Could you check a few things on this model? Use its own coordinates, in mm. Face numbers are marked on the shaded views. A direction names the side the tool comes from. Give positions to 0.01 mm unless a question says otherwise; leave off trailing zeros. Loops run counter-clockwise (first coordinate to the right, second up) from the corner with the lowest first, then second, coordinate; pieces in that order, holes last. Notation, with made-up numbers: (52, -1.5) - (97, -1.5) arc R20 cw to (97, 11.5) - close; hole circle Ø4 at (75.5, -20). An arc over 180 degrees is marked (long way). Write each question's results on one line, items separated by ' | '. Start each with the question number.
1) I want a section at D-D, the plane z = -22.75. Write out the boundary of the cut face in (x, y), and give its area (3 significant figures).
2) I want a section at A-A, the plane x = 25. Write out the boundary of the cut face in (y, z).
3) If we mould it in two halves opening along Z, with no side actions, what happens to the marked faces 1, 2 and 3? For each: +Z half, -Z half, draft (parallel to the pull), parting line (faces both ways), or undercut.
4) If I drill on probe 1 along X at (y, z) = (1.85, -7.5); probe 2 along X at (y, z) = (1.7, -6); probe 3 along Z at (x, y) = (4, 0.6), over which ranges is the centre line in solid material (lowest first)? Write a range as [from, to].
5) On a 3-axis mill with a long thin cutter (end or side, diameter ignored), from which of +Z, -Z, +X, -X, +Y, -Y can I reach the whole of each face in a straight line? I mean the marked faces 4 and 5. Say none if no direction works.
6) I want a section at B-B, the plane z = -17.5. Write out the boundary of the cut face in (x, y), and give its area (3 significant figures).
7) I want a section at C-C, the plane y = 1.55. Write out the boundary of the cut face in (x, z).
from build123d import *

# Parameters (mm, degrees)
SKETCH1_W           = 50
SKETCH1_H           = 25
SKETCH1_R           = 1.75
BOSS_EXTRUDE1_DEPTH = 3
SKETCH2_R           = 10
SKETCH2_W           = 10
SKETCH2_H           = 3
CUT_EXTRUDE1_DEPTH  = 10
FILLET1_R           = 5


with BuildPart() as part:
    # Sketch1 → Boss-Extrude1 (new body)
    with BuildSketch(Plane(origin=(0, 0, 0), x_dir=(1, 0, 0), z_dir=(0, 1, 0))):
        with Locations((25, 12.5)):
            Rectangle(SKETCH1_W, SKETCH1_H)
        with Locations(Location((25, 17.5, 0), (0, 0, 270))):
            Circle(SKETCH1_R, mode=Mode.SUBTRACT)
        with Locations(Location((25, 7.5, 0), (0, 0, 270))):
            Circle(SKETCH1_R, mode=Mode.SUBTRACT)
        with Locations(Location((5.463236706, 17.5, 0), (0, 0, 270))):
            Circle(SKETCH1_R, mode=Mode.SUBTRACT)
        with Locations(Location((5.463236706, 7.5, 0), (0, 0, 270))):
            Circle(SKETCH1_R, mode=Mode.SUBTRACT)
        with Locations(Location((44.777570027, 7.5, 0), (0, 0, 270))):
            Circle(SKETCH1_R, mode=Mode.SUBTRACT)
        with Locations(Location((44.777570027, 17.5, 0), (0, 0, 270))):
            Circle(SKETCH1_R, mode=Mode.SUBTRACT)
    extrude(amount=BOSS_EXTRUDE1_DEPTH)

    # Sketch2 → Cut-Extrude1 (cut)
    with BuildSketch(Plane(origin=(0, 3, 0), x_dir=(1, 0, 0), z_dir=(0, 1, 0))):
        with Locations((25, 32)):
            Circle(SKETCH2_R)
        with Locations((5, 23.5)):
            Rectangle(SKETCH2_W, SKETCH2_H)
        with Locations((45, 23.5)):
            Rectangle(SKETCH2_W, SKETCH2_H)
    extrude(amount=-CUT_EXTRUDE1_DEPTH, mode=Mode.SUBTRACT)

    # Fillet1
    # the kernel refuses this fillet: 5 mm, written as the material it takes off along each edge
    with BuildSketch(Plane(origin=(50, -12.5, 0), x_dir=(-1, 0, 0), z_dir=(0, 1, 0)), Plane(origin=(0, 15.5, -22), x_dir=(0, 0, 1), z_dir=(0, -1, 0))) as fillet1_piece_1:
        with BuildLine():
            CenterArc((FILLET1_R, -FILLET1_R), FILLET1_R, 90, 90)
            Line((0, -FILLET1_R), (-FILLET1_R * 0.02, -FILLET1_R))
            Line((-FILLET1_R * 0.02, -FILLET1_R), (-FILLET1_R * 0.02, FILLET1_R * 0.02))
            Line((-FILLET1_R * 0.02, FILLET1_R * 0.02), (FILLET1_R, FILLET1_R * 0.02))
            Line((FILLET1_R, FILLET1_R * 0.02), (FILLET1_R, 0))
        make_face()
    extrude(amount=28, mode=Mode.SUBTRACT)
    with BuildSketch(Plane(origin=(0, -12.5, 0), x_dir=(1, 0, 0), z_dir=(0, 1, 0)), Plane(origin=(50, 15.5, -22), x_dir=(0, 0, 1), z_dir=(0, -1, 0))) as fillet1_piece_2:
        with BuildLine():
            CenterArc((FILLET1_R, FILLET1_R), FILLET1_R, 180, 90)
            Line((0, FILLET1_R), (-FILLET1_R * 0.02, FILLET1_R))
            Line((-FILLET1_R * 0.02, FILLET1_R), (-FILLET1_R * 0.02, -FILLET1_R * 0.02))
            Line((-FILLET1_R * 0.02, -FILLET1_R * 0.02), (FILLET1_R, -FILLET1_R * 0.02))
            Line((FILLET1_R, -FILLET1_R * 0.02), (FILLET1_R, 0))
        make_face()
    extrude(amount=28, mode=Mode.SUBTRACT)
    with BuildSketch(Plane(origin=(40, 14.456439237, -25), x_dir=(-1, 0, 0), z_dir=(0, -1, 0))) as fillet1_piece_3:
        with BuildLine():
            CenterArc((4.582575695, -5), FILLET1_R, 90, 66.421821522)
            Line((0, -3), (-0.091651514, -2.96))
            ThreePointArc((-0.091651514, -2.96), (-0.1, -1.5), (-0.1, 0))
            Line((-0.1, 0), (0, 0.1))
            Line((0, 0.1), (4.582575695, 0.1))
            Line((4.582575695, 0.1), (4.582575695, 0))
        make_face()
    extrude(amount=25.912878475, mode=Mode.SUBTRACT)
    with BuildSketch(Plane(origin=(10, 14.456439237, -25), x_dir=(0, 0, 1), z_dir=(0, -1, 0))) as fillet1_piece_4:
        with BuildLine():
            CenterArc((5, -4.582575695), FILLET1_R, 113.578178478, 66.421821522)
            Line((0, -4.582575695), (-0.1, -4.582575695))
            Line((-0.1, -4.582575695), (-0.1, 0))
            Line((-0.1, 0), (0, 0.1))
            ThreePointArc((0, 0.1), (1.5, 0.1), (2.96, 0.091651514))
            Line((2.96, 0.091651514), (3, 0))
        make_face()
    extrude(amount=25.912878475, mode=Mode.SUBTRACT)
    with BuildSketch(Plane(origin=(17.858571571, -4.646428929, -25), x_dir=(-1, 0, 0), z_dir=(0, 1, 0))) as fillet1_piece_5:
        with BuildLine():
            CenterArc((1.858571571, 5), FILLET1_R, 233.130102354, 36.869897646)
            Line((-1.141428429, 1), (-1.201428429, 0.92))
            ThreePointArc((-1.201428429, 0.92), (-0.617614973, 0.446466141), (-0.071414284, -0.07))
            Line((-0.071414284, -0.07), (0, -0.1))
            Line((0, -0.1), (1.858571571, -0.1))
            Line((1.858571571, -0.1), (1.858571571, 0))
        make_face()
    extrude(amount=12.292857857, mode=Mode.SUBTRACT)
    with BuildSketch(Plane(origin=(32.141428429, -4.646428929, -25), x_dir=(-0.7521682970876359, 0, 0.658971056159742), z_dir=(0, 1, 0))) as fillet1_piece_6:
        with BuildLine():
            CenterArc((1.896896667, 4.985586357), FILLET1_R, 228.778553177, 36.869897646)
            Line((-1.397958614, 1.224744871), (-1.46385572, 1.149528042))
            Line((-1.46385572, 1.149528042), (-0.065897106, -0.07521683))
            Line((-0.065897106, -0.07521683), (0.007587587, -0.099711727))
            ThreePointArc((0.007587587, -0.099711727), (0.758758667, -0.071172714), (1.509929747, -0.099711727))
            Line((1.509929747, -0.099711727), (1.517517334, 0))
        make_face()
    extrude(amount=12.292857857, mode=Mode.SUBTRACT)


solid = part.part
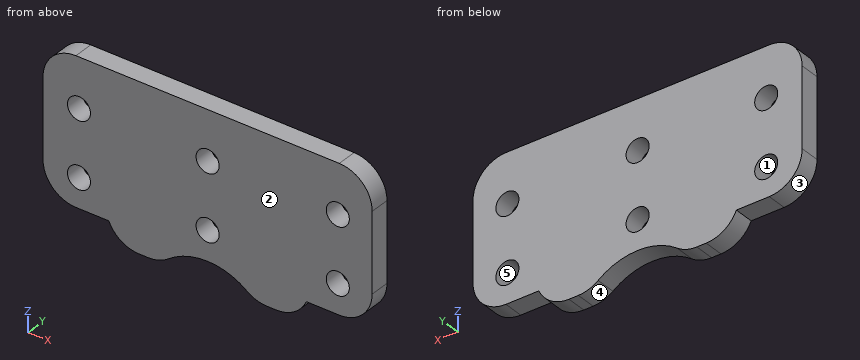
Answers:
1) outline: (10.41, 0) - (21.2, 0) - (21.2, 3) - (10.41, 3) - close; (28.8, 0) - (39.59, 0) - (39.59, 3) - (28.8, 3) - close | area: 64.8 mm2
2) outline: (0, -22) - (3, -22) - (3, -19.25) - (0, -19.25) - close; (0, -15.75) - (3, -15.75) - (3, -9.25) - (0, -9.25) - close; (0, -5.75) - (3, -5.75) - (3, 0) - (0, 0) - close
3) face 1: undercut | face 2: draft | face 3: -Z half
4) probe 1: x = [0, 3.71], [7.21, 23.25], [26.75, 43.03], [46.53, 50] | probe 2: x = [0, 4.56], [6.36, 24.1], [25.9, 43.88], [45.68, 50] | probe 3: z = [-21.9, -18.46], [-16.54, -8.46], [-6.54, -0.1]
5) face 4: -Z, +Y, -Y | face 5: +Y, -Y
6) outline: (0.03, 0) - (3.71, 0) - (3.71, 3) - (0.03, 3) - close; (7.21, 0) - (23.25, 0) - (23.25, 3) - (7.21, 3) - close; (26.75, 0) - (43.03, 0) - (43.03, 3) - (26.75, 3) - close; (46.53, 0) - (49.97, 0) - (49.97, 3) - (46.53, 3) - close | area: 118 mm2
7) outline: (0, -17) arc R5 ccw to (5, -22) - (10, -22) arc R5 ccw to (14.58, -25) - (16, -25) arc R5 ccw to (19, -24) arc R10 cw to (31, -24) arc R5 ccw to (34, -25) - (35.42, -25) arc R5 ccw to (40, -22) - (45, -22) arc R5 ccw to (50, -17) - (50, -5) arc R5 ccw to (45, 0) - (5, 0) arc R5 ccw to (0, -5) - close; hole circle Ø3.5 at (5.46, -17.5); hole circle Ø3.5 at (5.46, -7.5); hole circle Ø3.5 at (25, -17.5); hole circle Ø3.5 at (25, -7.5); hole circle Ø3.5 at (44.78, -17.5); hole circle Ø3.5 at (44.78, -7.5)
